```python
from build123d import *

# Parameters (mm, degrees)
BOSS_EXTRUDE3_DEPTH = 50.8
SKETCH3_R           = 44.45
CUT_EXTRUDE1_DEPTH  = 5.08


with BuildPart() as part:
    # Sketch2 → Boss-Extrude3 (new body)
    with BuildSketch(Plane(origin=(0, 0, 0), x_dir=(1, 0, 0), z_dir=(0, 1, 0))):
        with BuildLine():
            Line((828.937277778, 239.610630395), (-828.937277778, 239.610630395))
            add(Edge.make_bspline(
                [(-828.937277778, 239.610630395), (-830.5402629, 239.610630395), (-833.790113095, 238.979161906), (-837.861109298, 236.262109298), (-840.578161906, 232.191113095), (-841.209630395, 228.9412629), (-841.209630395, 227.338277778)],
                knots=[-0.770319033, -0.770319033, -0.770319033, -0.770319033, -0.385159516, 0, 0.385159516, 0.770319033, 0.770319033, 0.770319033, 0.770319033], degree=3))
            Line((-841.209630395, 227.338277778), (-841.209630395, -227.338277778))
            add(Edge.make_bspline(
                [(-841.209630395, -227.338277778), (-841.209630395, -228.9412629), (-840.578161906, -232.191113095), (-837.861109298, -236.262109298), (-833.790113095, -238.979161906), (-830.5402629, -239.610630395), (-828.937277778, -239.610630395)],
                knots=[-0.770319033, -0.770319033, -0.770319033, -0.770319033, -0.385159516, 0, 0.385159516, 0.770319033, 0.770319033, 0.770319033, 0.770319033], degree=3))
            Line((-828.937277778, -239.610630395), (828.937277778, -239.610630395))
            add(Edge.make_bspline(
                [(828.937277778, -239.610630395), (830.5402629, -239.610630395), (833.790113095, -238.979161906), (837.861109298, -236.262109298), (840.578161906, -232.191113095), (841.209630395, -228.9412629), (841.209630395, -227.338277778)],
                knots=[-0.770319033, -0.770319033, -0.770319033, -0.770319033, -0.385159516, 0, 0.385159516, 0.770319033, 0.770319033, 0.770319033, 0.770319033], degree=3))
            Line((841.209630395, -227.338277778), (841.209630395, 227.338277778))
            add(Edge.make_bspline(
                [(841.209630395, 227.338277778), (841.209630395, 228.9412629), (840.578161906, 232.191113095), (837.861109298, 236.262109298), (833.790113095, 238.979161906), (830.5402629, 239.610630395), (828.937277778, 239.610630395)],
                knots=[-0.770319033, -0.770319033, -0.770319033, -0.770319033, -0.385159516, 0, 0.385159516, 0.770319033, 0.770319033, 0.770319033, 0.770319033], degree=3))
        make_face()
        with BuildLine():
            Line((183, 5), (719.067867535, 84.701940777))
            ThreePointArc((719.067867535, 84.701940777), (734.37520483, 87.746759477), (747.352138783, 96.41766953))
            Line((747.352138783, 96.41766953), (805.740119782, 154.805650529))
            ThreePointArc((805.740119782, 154.805650529), (811.568721914, 170.02928211), (804.130185735, 184.534444667))
            ThreePointArc((804.130185735, 184.534444667), (764.162148174, 206.781275976), (719.074, 214.489999861))
            Line((719.074, 214.489999861), (97, 183))
            Line((97, 183), (-97, 183))
            Line((-97, 183), (-744.729609, 176.382687101))
            ThreePointArc((-744.729609, 176.382687101), (-774.626285266, 163.729853371), (-786.973045304, 133.705480442))
            Line((-786.973045304, 133.705480442), (-786.865578677, -19.509544471))
            ThreePointArc((-786.865578677, -19.509544471), (-772.505899638, -51.439554767), (-739.089614065, -61.883586467))
            Line((-739.089614065, -61.883586467), (-183, 5))
            Line((-183, 5), (-183, -5))
            Line((-183, -5), (-757.976293163, -88.338177387))
            ThreePointArc((-757.976293163, -88.338177387), (-811.160134278, -154.450903881), (-749.042879972, -212.251079294))
            Line((-749.042879972, -212.251079294), (-97, -183))
            Line((-97, -183), (97, -183))
            Line((97, -183), (751.749025656, -224.140342752))
            ThreePointArc((751.749025656, -224.140342752), (797.345746833, -187.130639885), (764.1784404, -138.667160105))
            Line((764.1784404, -138.667160105), (183, -5))
            Line((183, -5), (183, 5))
        make_face(mode=Mode.SUBTRACT)
    extrude(amount=BOSS_EXTRUDE3_DEPTH)

    # Sketch3 → Cut-Extrude1 (cut)
    with BuildSketch(Plane.XZ):
        with Locations((754.506388348, 181.844577047)):
            Circle(SKETCH3_R)
        with BuildLine():
            Line((820.56615944, -139.979610872), (762.17817844, -81.591629872))
            ThreePointArc((762.17817844, -81.591629872), (719.067867535, -63.734754417), (675.95755663, -81.591629872))
            Line((675.95755663, -81.591629872), (617.569575631, -139.979610872))
            ThreePointArc((617.569575631, -139.979610872), (605.630504143, -171.163078474), (620.867299038, -200.874863358))
            ThreePointArc((620.867299038, -200.874863358), (719.067867535, -235.45718636), (817.268436033, -200.874863358))
            ThreePointArc((817.268436033, -200.874863358), (832.505230927, -171.163078474), (820.56615944, -139.979610872))
        make_face()
    extrude(amount=-CUT_EXTRUDE1_DEPTH, mode=Mode.SUBTRACT)


solid = part.part
```
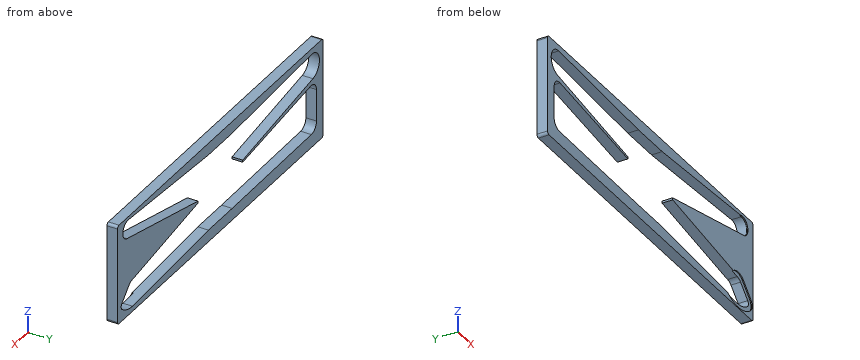
CAD build for the part. Positions are in the model's coordinates, mm. Coordinates: 2 decimals unless noted, no trailing zeros. Write each loop counter-clockwise with the first axis right and the second up, starting at its lowest first coordinate (ties: lowest second). Pieces come first, ordered by that corner, then holes. Notation, with made-up numbers: (13.5, -10.5) -> (24.5, -10.5) arc R24 cw to (24.5, 16.5) -> close; hole circle Ø8 at (-31, 82.5). An arc over 180 degrees is marked (long way). Return JSON: item names as keys, results as strings. Group by question number.
Q1. Cut at D-D, the plane z = -119. Give the cut face in (x, y), then the cut area to 3 significant figures.
Q2. Drill centre lines: line 1 (Z direction, x = -231, y = 9); line 2 (Z direction, x = 414, y = 47.5); line 3 (Z direction, x = 18.5, y = 32). Where is each one in solid material? Low to high.
Q3. Cut at A-A, the plane x = 12. Give the cut face in (y, z).
Q4. Cut at C-C, the plane x = 558.5. Give the cut face in (y, z), then the cut area to 3 significant figures.
Q5. Cut at B-B, the plane z = 116. Give the cut face in (x, y).
Returned:
{
 "1": {"outline": "(-841.21, 0) -> (-786.96, 0) -> (-786.96, 50.8) -> (-841.21, 50.8) -> close; (769.93, 5.08) -> (799.59, 5.08) -> (799.59, 0) -> (841.21, 0) -> (841.21, 50.8) -> (769.93, 50.8) -> close", "area": "6,230 mm2"},
 "2": {"line 1": "z = -239.61 to -181.63, 0.77 to 11.96, 189.01 to 239.61", "line 2": "z = -239.61 to -199.05, -39.34 to 58.13, 202.92 to 239.61", "line 3": "z = -239.61 to -183, 183 to 239.61"},
 "3": {"outline": "(0, -239.61) -> (50.8, -239.61) -> (50.8, -183) -> (0, -183) -> close; (0, 183) -> (50.8, 183) -> (50.8, 239.61) -> (0, 239.61) -> close"},
 "4": {"outline": "(0, -239.61) -> (50.8, -239.61) -> (50.8, -206.36) -> (0, -206.36) -> close; (0, -60.83) -> (50.8, -60.83) -> (50.8, 91.36) -> (0, 91.36) -> close; (0, 212) -> (50.8, 212) -> (50.8, 239.61) -> (0, 239.61) -> close", "area": "10,800 mm2"},
 "5": {"outline": "(-841.21, 0) -> (-801.24, 0) -> (-801.24, 50.8) -> (-841.21, 50.8) -> close; (665.62, 0) -> (841.21, 0) -> (841.21, 50.8) -> (665.62, 50.8) -> close"}
}
